Design review of the part shown in the three views and the two pictorial views. Dimensions are in mm from the part's minimum x, y and z. Round coordinates to 2 decimals unless told otherwise and drop trailing zeros. Loops run counter-clockwise (first coordinate to the right, second up) from the corner with the lowest first, then second, coordinate; pieces in that order, holes last. Notation, with made-up numbers: (-18.75, -24) -> (7.25, -24) arc R6 ccw to (7.25, -19) -> close; hole circle Ø7 at (-24, -9.5). An arc over 180 degrees is marked (long way). Return JSON: item names as keys, results as strings. Group by question number.
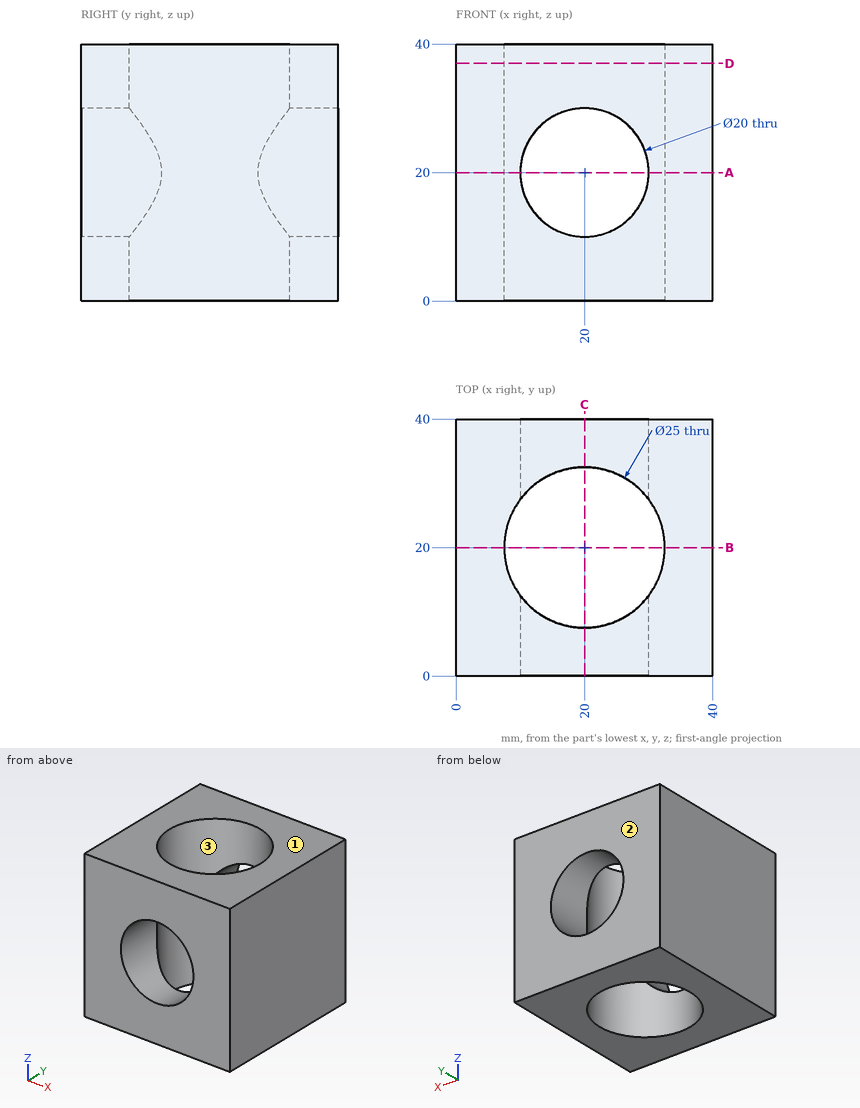
1. For P1, Ø6, axis at x = 11.5, y = 23, coming from the -Z side, flat-tipped, find the tip position at first contact; note if it passes through.
2. We need section B-B, the plane y = 20. Write out the cut boundary in (x, z).
3. We need section A-A, the plane z = 20. Write out the cut boundary in (x, y).
4. We need section C-C, the plane x = 20. Write out the cut boundary in (y, z), then the cut area to 3 significant figures.
5. Wall thickness on line 1 (Z direction, x = 20, y = 3); line 2 (X direction, y = 19.5, z = 34): over which ranges is each line inside the solid? List them lowest first.
6. Draft analysis for pull direction Y (two halves, no side actions). For the marked faces 1, 2 and 3, state which applies: pulls with the +Y half, pulls with the -Y half, needs draft (parallel to the pull), parting line crosses it, or undercut.
7. We need section D-D, the plane z = 37. Write out the cut boundary in (x, y).
Check sheet entries:
{
 "1": {"P1": "passes through"},
 "2": {"outline": "(0, 0) -> (7.5, 0) -> (7.5, 40) -> (0, 40) -> close; (32.5, 0) -> (40, 0) -> (40, 40) -> (32.5, 40) -> close"},
 "3": {"outline": "(0, 0) -> (10, 0) -> (10, 12.5) arc R12.5 cw to (10, 27.5) -> (10, 40) -> (0, 40) -> close; (30, 0) -> (40, 0) -> (40, 40) -> (30, 40) -> (30, 27.5) arc R12.5 cw to (30, 12.5) -> close"},
 "4": {"outline": "(0, 0) -> (7.5, 0) -> (7.5, 10) -> (0, 10) -> close; (0, 30) -> (7.5, 30) -> (7.5, 40) -> (0, 40) -> close; (32.5, 0) -> (40, 0) -> (40, 10) -> (32.5, 10) -> close; (32.5, 30) -> (40, 30) -> (40, 40) -> (32.5, 40) -> close", "area": "300 mm²"},
 "5": {"line 1": "z = 0 to 10, 30 to 40", "line 2": "x = 0 to 7.51, 32.49 to 40"},
 "6": {"face 1": "needs draft", "face 2": "pulls with the +Y half", "face 3": "undercut"},
 "7": {"outline": "(0, 0) -> (40, 0) -> (40, 40) -> (0, 40) -> close; hole circle Ø25 at (20, 20)"}
}
